Build history of the part. All positions in model axes, mm. Face numbers are marked on the shaded views. A direction names the side the tool comes from. Coordinates: 2 decimals unless noted, no trailing zeros. Order: outer loops, then holes, each group sorted by start corner. A loop starts at its lowest first (then second) coordinate and runs counter-clockwise, first axis right, second up. Notation, with made-up numbers: (51, -32) - (76, -32) arc R21 cw to (76, 5) - close; hole circle Ø3 at (52.25, -27). An arc over 180 degrees is marked (long way). Return JSON: item names as keys, results as strings.
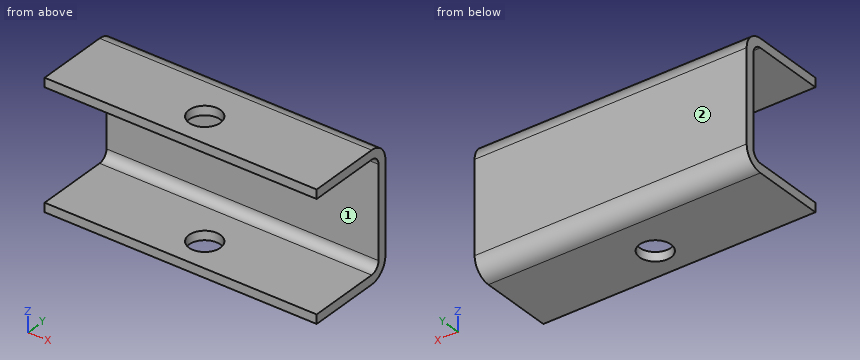
from build123d import *

# Parameters (mm, degrees)
SKETCH1_W                         = 76.2
SKETCH1_H                         = 35.75
BASE_FLANGE1_DEPTH                = 2.54
EDGE_FLANGE1_STRIP_W              = 15.24
EDGE_FLANGE1_STRIP_H              = 2.54
EDGE_FLANGE1_STRIP_CUT_DEPTH      = 76.2
EDGE_FLANGE1_STRIP_2_W            = 15.24
EDGE_FLANGE1_STRIP_2_H            = 2.54
EDGE_FLANGE1_STRIP_CUT_2_DEPTH    = 76.2
EDGE_FLANGE1_DEPTH                = 76.2
EDGE_FLANGE1_BEND_DEPTH           = 76.2
TAP_DRILL_FOR_M10X1_25_TAP1_D     = 8.8
TAP_DRILL_FOR_M10X1_25_TAP1_DEPTH = 35.75
TAP_DRILL_FOR_M10X1_25_TAP1_TIP   = 2.643786724


# Sheet-metal steps are written as plain solids
with BuildPart() as part:
    # Sketch1 → Base-Flange1 (new body)
    with BuildSketch(Plane(origin=(0, 0, 0), x_dir=(1, 0, 0), z_dir=(0, 1, 0))):
        with Locations((37.147058824, -17.382352941)):
            Rectangle(SKETCH1_W, SKETCH1_H)
    extrude(amount=-BASE_FLANGE1_DEPTH)

    # Edge-Flange1 strip (across the edge) → Edge-Flange1 strip cut (cut)
    with BuildSketch(Plane(origin=(75.247058824, -2.54, 35.257352941), x_dir=(0, 0, -1), z_dir=(-1, 0, 0))):
        with Locations((-2.54, -1.27)):
            Rectangle(EDGE_FLANGE1_STRIP_W, EDGE_FLANGE1_STRIP_H)
    extrude(amount=EDGE_FLANGE1_STRIP_CUT_DEPTH, mode=Mode.SUBTRACT)

    # Edge-Flange1 strip 2 (across the edge) → Edge-Flange1 strip cut 2 (cut)
    with BuildSketch(Plane(origin=(-0.952941176, -2.54, -0.492647059), x_dir=(0, 0, 1), z_dir=(1, 0, 0))):
        with Locations((-2.54, -1.27)):
            Rectangle(EDGE_FLANGE1_STRIP_2_W, EDGE_FLANGE1_STRIP_2_H)
    extrude(amount=EDGE_FLANGE1_STRIP_CUT_2_DEPTH, mode=Mode.SUBTRACT)

    # Edge-Flange1 section (across the edge) → Edge-Flange1 (add)
    with BuildSketch(Plane(origin=(75.247058824, -2.54, 35.257352941), x_dir=(0, 0, -1), z_dir=(-1, 0, 0))):
        with BuildLine():
            Line((0, 2.54), (0, 22.86))
            Line((0, 22.86), (2.54, 22.86))
            Line((2.54, 22.86), (2.54, 2.54))
            ThreePointArc((2.54, 2.54), (3.283948776, 0.743948776), (5.08, 0))
            Line((5.08, 0), (5.08, -2.54))
            ThreePointArc((5.08, -2.54), (1.487897552, -1.052102448), (0, 2.54))
        make_face()
    extrude(amount=EDGE_FLANGE1_DEPTH)

    # Edge-Flange1 section 2 (across the edge) → Edge-Flange1 bend (add)
    with BuildSketch(Plane(origin=(-0.952941176, -2.54, -0.492647059), x_dir=(0, 0, 1), z_dir=(1, 0, 0))):
        with BuildLine():
            Line((0, 2.54), (0, 22.86))
            Line((0, 22.86), (2.54, 22.86))
            Line((2.54, 22.86), (2.54, 2.54))
            ThreePointArc((2.54, 2.54), (3.283948776, 0.743948776), (5.08, 0))
            Line((5.08, 0), (5.08, -2.54))
            ThreePointArc((5.08, -2.54), (1.487897552, -1.052102448), (0, 2.54))
        make_face()
    extrude(amount=EDGE_FLANGE1_BEND_DEPTH)

    # Tap Drill for M10x1.25 Tap1
    with Locations(Plane.XY.offset(35.257352941)):
        with Locations((37.147058824, -16.51)):
            Hole(TAP_DRILL_FOR_M10X1_25_TAP1_D / 2, depth=TAP_DRILL_FOR_M10X1_25_TAP1_DEPTH)
            with Locations((0, 0, -(TAP_DRILL_FOR_M10X1_25_TAP1_DEPTH + TAP_DRILL_FOR_M10X1_25_TAP1_TIP / 2))):  # 118° drill point
                Cone(0, TAP_DRILL_FOR_M10X1_25_TAP1_D / 2, TAP_DRILL_FOR_M10X1_25_TAP1_TIP, mode=Mode.SUBTRACT)


solid = part.part
1. Cut at B-B on x = 32. Give the cut face in (y, z).
Check values:
{"outline": "(-25.4, -0.49) - (-5.08, -0.49) arc R5.08 ccw to (0, 4.59) - (0, 30.18) arc R5.08 ccw to (-5.08, 35.26) - (-25.4, 35.26) - (-25.4, 32.72) - (-5.08, 32.72) arc R2.54 cw to (-2.54, 30.18) - (-2.54, 4.59) arc R2.54 cw to (-5.08, 2.05) - (-25.4, 2.05) - close"}
2. Cut at C-C on y = -7. Give the cut face in (x, z).
Check values:
{"outline": "(-0.95, -0.49) - (75.25, -0.49) - (75.25, 2.05) - (-0.95, 2.05) - close; (-0.95, 32.72) - (75.25, 32.72) - (75.25, 35.26) - (-0.95, 35.26) - close"}
3. Cut at A-A on y = -16.51. Give the cut face in (x, z).
Check values:
{"outline": "(-0.95, -0.49) - (32.75, -0.49) - (32.75, 2.05) - (-0.95, 2.05) - close; (-0.95, 32.72) - (32.75, 32.72) - (32.75, 35.26) - (-0.95, 35.26) - close; (41.55, -0.49) - (75.25, -0.49) - (75.25, 2.05) - (41.55, 2.05) - close; (41.55, 32.72) - (75.25, 32.72) - (75.25, 35.26) - (41.55, 35.26) - close"}
4. Cut at D-D on z = 33.5. Give the cut face in (x, y), plus the area to 3 significant figures.
Check values:
{"outline": "(-0.95, -25.4) - (75.25, -25.4) - (75.25, -1.24) - (-0.95, -1.24) - close; hole circle Ø8.8 at (37.15, -16.51)", "area": "1,780 mm²"}
5. Probe L1, parallel to Z at x = 49, y = -22.25; L2, parallel to X at y = -16.51, z = 0.65; L3, parallel to Y at x = 30, z = 18.5. List the from-to ranges inside material, lowest first.
Check values:
{"L1": "-0.49 to 2.05, 32.72 to 35.26", "L2": "-0.95 to 32.75, 41.55 to 75.25", "L3": "-2.54 to 0"}
6. Tool access for the marked faces 1 and 2: list every direction of +Z, -Z, +X, -X, +Y, -Y with a clear straight run to the whole face (end or side of a thin tool).
Check values:
{"face 1": "+X, -X, -Y", "face 2": "+Z, -Z, +X, -X, +Y"}
7. Drop flat-ended pins along their axis: pin 1 (1 mm diameter, centred on x = 32, y = -3.5, fed in from -Z); pin 2 (4 mm diameter, centred on x = 58.5, z = 29, fed in from -Y); pin 3 (6 mm diameter, centred on x = 57.5, z = 25, fed in from -Y). Give the stop position or say it passes through.
Check values:
{"pin 1": "z = -0.38", "pin 2": "y = -2.68", "pin 3": "y = -2.54"}
